Read the model definition and answer for the solid it produces. Units are mm, in the model's axes. Face numbers are marked on the shaded views. A direction names the side the tool comes from. Coordinates: 2 decimals unless noted, no trailing zeros. Loops run counter-clockwise (first coordinate to the right, second up) from the corner with the lowest first, then second, coordinate; pieces in that order, holes last. Notation, with made-up numbers: M -3.75,8 L 27.25,8 A15 cw 27.25,32 Z; hole C -33.75,32.5 d11. An arc over 180 degrees is marked long. One line per item, written item: value. Start each with the question number.
1. Flat-ended cylindrical pins translate along their axes: pin 1 (12 mm diameter, centred on x = 9, z = -7, fed in from -Y); pin 2 (5 mm diameter, centred on x = -5.5, y = 7.5, fed in from +Z); pin 3 (4 mm diameter, centred on x = 12.5, y = 5, fed in from +Z); pin 4 (12 mm diameter, centred on x = -10, z = 0, fed in from +Y). Find the tip coordinate at first contact, or state that the pin passes through.
2. The part is cut by section D-D (z = -11). Write down the section's boundary in (x, y).
3. The part is cut by section C-C (x = -1). Write down the section's boundary in (y, z).
4. For the marked faces 1, 2 and 3, determine the directions among +Z, -Z, +X, -X, +Y, -Y from which every point of the face is accessible in a straight line to the end or side of a thin tool.
5. Consider probe 1 along Y at (x, z) = (15, -18); probe 2 along Z at (x, y) = (16.5, 19); probe 3 along Y at (x, z) = (-8, 2). Determine where each line is inside the solid, lowest interval first.
6. The part is cut by section A-A (x = -10.5). Write down the section's boundary in (y, z).
7. The part is cut by section B-B (z = 7). Write down the section's boundary in (x, y), then the cut area to 4 significant figures.
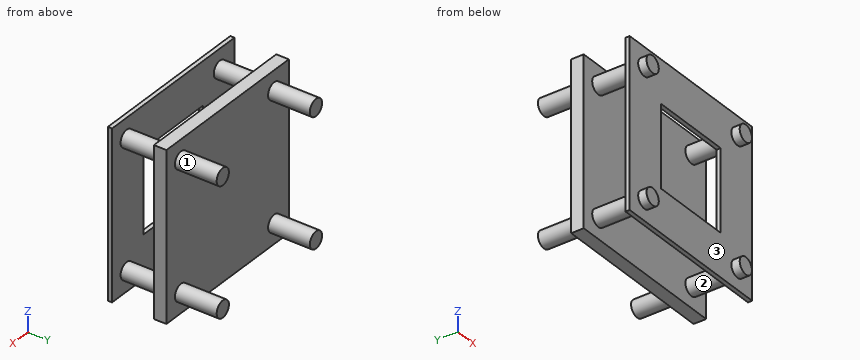
```python
from build123d import *

# Parameters (mm, degrees)
SKETCH_2_W          = 40
SKETCH_2_H          = 40
EXTRUDE_2_DEPTH     = 1
SKETCH_3_R          = 2
CUT_EXTRUDE_1_DEPTH = 3
EXTRUDE_START       = 10
SKETCH_9_W          = 40
SKETCH_9_H          = 40
EXTRUDE_4_DEPTH     = 3
SKETCH_3_3_R        = 2
EXTRUDE_5_DEPTH     = 24
EXTRUDE_START_2     = -2
SKETCH_2_8_R        = 2
EXTRUDE_6_DEPTH     = 2
SKETCH_2_9_W        = 19.5
SKETCH_2_9_H        = 19.5
CUT_EXTRUDE_2_DEPTH = 10


with BuildPart() as part:
    # Sketch 2 → Extrude 2 (new body)
    with BuildSketch(Plane(origin=(0, 0, 0), x_dir=(1, 0, 0), z_dir=(0, 1, 0))):
        Rectangle(SKETCH_2_W, SKETCH_2_H)
    extrude(amount=EXTRUDE_2_DEPTH)

    # Sketch 3 → Cut-Extrude 1 (cut)
    with BuildSketch(Plane(origin=(0, 0, 0), x_dir=(1, 0, 0), z_dir=(0, 1, 0))):
        with Locations(Location((-15.224798987, -15.224798987, 0), (0, 0, 270))):
            Circle(SKETCH_3_R)
        with Locations(Location((15.224798987, -15.224798987, 0), (0, 0, 270))):
            Circle(SKETCH_3_R)
        with Locations(Location((15.224798987, 15.224798987, 0), (0, 0, 270))):
            Circle(SKETCH_3_R)
        with Locations(Location((-15.224798987, 15.224798987, 0), (0, 0, 270))):
            Circle(SKETCH_3_R)
    extrude(amount=CUT_EXTRUDE_1_DEPTH, mode=Mode.SUBTRACT)



with BuildPart() as body_2:
    # Sketch 9 → Extrude 4 (new body)
    with BuildSketch(Plane(origin=(0, 1, 0), x_dir=(1, 0, 0), z_dir=(0, 1, 0)).offset(EXTRUDE_START)):
        Rectangle(SKETCH_9_W, SKETCH_9_H)
    extrude(amount=EXTRUDE_4_DEPTH)

    # Sketch 3_3 → Extrude 5 (add)
    with BuildSketch(Plane(origin=(0, 0, 0), x_dir=(1, 0, 0), z_dir=(0, 1, 0))):
        with Locations(Location((-15.224798987, -15.224798987, 0), (0, 0, 270))):
            Circle(SKETCH_3_3_R)
        with Locations(Location((15.224798987, -15.224798987, 0), (0, 0, 270))):
            Circle(SKETCH_3_3_R)
        with Locations(Location((15.224798987, 15.224798987, 0), (0, 0, 270))):
            Circle(SKETCH_3_3_R)
        with Locations(Location((-15.224798987, 15.224798987, 0), (0, 0, 270))):
            Circle(SKETCH_3_3_R)
    extrude(amount=EXTRUDE_5_DEPTH)


with BuildPart() as part_1:
    add(part.part)

    add(body_2.part)  # Extrude 6 merges body 2
    # Sketch 2_8 → Extrude 6 (add)
    with BuildSketch(Plane(origin=(0, 0, 0), x_dir=(1, 0, 0), z_dir=(0, 1, 0)).offset(EXTRUDE_START_2)):
        with Locations(Location((15.224798987, 15.224798987, 0), (0, 0, 270))):
            Circle(SKETCH_2_8_R)
        with Locations(Location((-15.224798987, -15.224798987, 0), (0, 0, 270))):
            Circle(SKETCH_2_8_R)
        with Locations(Location((15.224798987, -15.224798987, 0), (0, 0, 270))):
            Circle(SKETCH_2_8_R)
        with Locations(Location((-15.224798987, 15.224798987, 0), (0, 0, 270))):
            Circle(SKETCH_2_8_R)
    extrude(amount=EXTRUDE_6_DEPTH)

    # Sketch 2_9 → Cut-Extrude 2 (cut)
    with BuildSketch(Plane(origin=(0, 0, 0), x_dir=(1, 0, 0), z_dir=(0, 1, 0))):
        Rectangle(SKETCH_2_9_W, SKETCH_2_9_H)
    extrude(amount=CUT_EXTRUDE_2_DEPTH, mode=Mode.SUBTRACT)


solid = part_1.part
```
Answer block:
1. pin 1: stops at y = 0
1. pin 2: passes through
1. pin 3: stops at z = 17.09
1. pin 4: stops at y = 14
2. outline: M -20,0 L 20,0 L 20,1 L -20,1 Z; M -20,11 L 20,11 L 20,14 L -20,14 Z
3. outline: M 0,-20 L 1,-20 L 1,-9.75 L 0,-9.75 Z; M 0,9.75 L 1,9.75 L 1,20 L 0,20 Z; M 11,-20 L 14,-20 L 14,20 L 11,20 Z
4. face 1: +Y
4. face 2: none
4. face 3: -Y
5. probe 1: y = 0 to 1, 11 to 14
5. probe 2: z = -16.77 to -13.68, 13.68 to 16.77
5. probe 3: y = 11 to 14
6. outline: M 0,-20 L 1,-20 L 1,20 L 0,20 Z; M 11,-20 L 14,-20 L 14,20 L 11,20 Z
7. outline: M -20,0 L -9.75,0 L -9.75,1 L -20,1 Z; M -20,11 L 20,11 L 20,14 L -20,14 Z; M 9.75,0 L 20,0 L 20,1 L 9.75,1 Z
7. area: 140.5 mm2
